Geometry check sheet. Reference: the model listing, model coordinates, mm. Face numbers are marked on the shaded views. A direction names the side the tool comes from. Coordinates: 2 decimals unless noted, no trailing zeros. Write each loop counter-clockwise with the first axis right and the second up, starting at its lowest first coordinate (ties: lowest second). Pieces come first, ordered by that corner, then holes. Notation, with made-up numbers: M -28.75,66.5 L 22.25,66.5 A36 ccw 22.25,105.5 Z; hole C -27,36.5 d11. An arc over 180 degrees is marked long. Put each result on its own line as item: value. Start each with the question number.
1) Scan lines: line 1 along Y through (x, z) = (0.55, 1); line 2 along X through (y, z) = (-0.9, -3.25); line 3 along Y through (x, z) = (1.15, -1.5). Record each from-to range of solid material in increasing order.
2) Cross-section at A-A on z = -1.5. Record the cut outline in (x, y) (3 decimals).
3) Gauge pin test, flat ends, axial feed: pin 1 (2 mm diameter, centred on x = 0, y = -1.5, fed in from -Z); pin 2 (1 mm diameter, centred on x = -0.5, z = -2, fed in from +Y) (3 decimals); pin 3 (1 mm diameter, centred on x = -2, z = -2.5, fed in from +Y). Record the tip position at first contact, or that the pin passes through.
4) Set-up check for the marked faces 1 and 2: record each of +Z, -Z, +X, -X, +Y, -Y from which the full face is reachable in a straight line by a thin tool's end or side.
5) Cross-section at B-B on z = -4.25. Record the cut outline in (x, y).
from build123d import *

# Parameters (mm, degrees)
F0_R     = 2.75
F1_DEPTH = 3
F2_R     = 2
F3_R     = 2.475
F4_DEPTH = 5.5
F5_R     = 2.475


with BuildPart() as f1:
    # F0 (on Top) → F1 (new body)
    with BuildSketch(Plane.XY):
        Circle(F0_R)
    extrude(amount=F1_DEPTH)

    # F2
    f2_edges = [f1.edges().sort_by_distance(p)[0] for p in [
        (-2.75, 0, 3),
    ]]
    fillet(f2_edges, radius=F2_R)

    # F3 (on face) → F4 (join)
    with BuildSketch(Plane(origin=(0, 0, 0), x_dir=(1, 0, 0), z_dir=(0, 0, -1))):
        Circle(F3_R)
    extrude(amount=F4_DEPTH)

    # F5
    f5_edges = [f1.edges().sort_by_distance(p)[0] for p in [
        (-2.475, 0, -5.5),
    ]]
    fillet(f5_edges, radius=F5_R)


solid = f1.part
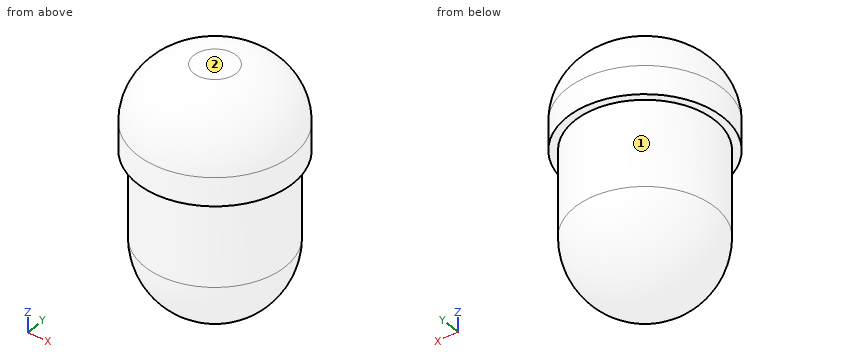
Answer key:
1. line 1: y = -2.69 to 2.69
1. line 2: x = -2.29 to 2.29
1. line 3: y = -2.19 to 2.19
2. outline: C 0,0 d4.95
3. pin 1: stops at z = -5.45
3. pin 2: stops at y = 2.475
3. pin 3: stops at y = 1.97
4. face 1: -Z
4. face 2: +Z, +X, -X, +Y, -Y
5. outline: C 0,0 d4.3
